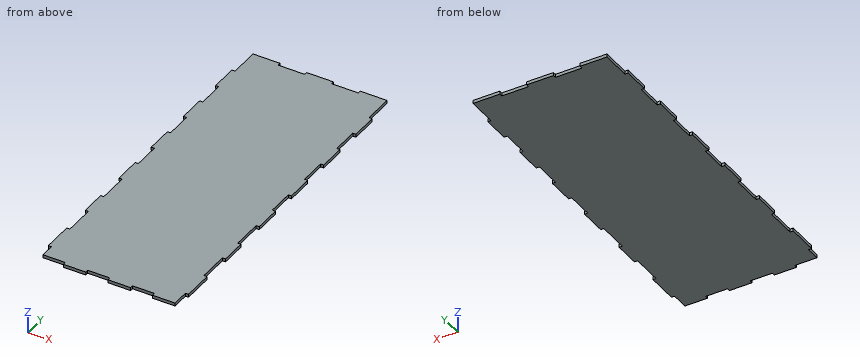
from build123d import *

# Parameters (mm, degrees)
BOSS_EXTRUDE1_DEPTH = 3


with BuildPart() as part:
    # Sketch1 → Boss-Extrude1 (new body)
    with BuildSketch(Plane.XY):
        Polygon((64.15, 153.019232641), (64.15, 178.481870793), (67.15, 178.481870793), (67.15, 204.244508944), (64.15, 204.244508944), (64.15, 229.707147096), (67.15, 229.707147096), (67.15, 255.469785247), (64.15, 255.469785247), (64.15, 280.932423398), (67.15, 280.932423398), (67.15, 306.69506155), (64.15, 306.69506155), (64.15, 335.261916889), (38.37, 335.261916889), (38.37, 332.261916889), (12.89, 332.261916889), (12.89, 335.261916889), (-12.89, 335.261916889), (-12.89, 332.261916889), (-38.37, 332.261916889), (-38.37, 335.261916889), (-64.15, 335.261916889), (-64.15, 306.69506155), (-67.15, 306.69506155), (-67.15, 280.932423398), (-64.15, 280.932423398), (-64.15, 255.469785247), (-67.15, 255.469785247), (-67.15, 229.707147096), (-64.15, 229.707147096), (-64.15, 204.244508944), (-67.15, 204.244508944), (-67.15, 178.481870793), (-64.15, 178.481870793), (-64.15, 153.019232641), (-67.15, 153.019232641), (-67.15, 127.25659449), (-64.15, 127.25659449), (-64.15, 98.12172779), (-67.15, 98.12172779), (-67.15, 73.67315636), (-64.15, 73.67315636), (-64.15, 44.27458493), (-67.15, 44.27458493), (-67.15, 14.8260135), (-64.15, 14.8260135), (-64.15, 1.5), (-42.916666667, 1.5), (-42.916666667, -1.5), (-21.383333333, -1.5), (-21.383333333, 1.5), (-0.15, 1.5), (-0.15, -1.5), (21.383333333, -1.5), (21.383333333, 1.5), (42.616666667, 1.5), (42.616666667, -1.5), (64.15, -1.5), (64.15, 14.8260135), (67.15, 14.8260135), (67.15, 44.27458493), (64.15, 44.27458493), (64.15, 73.67315636), (67.15, 73.67315636), (67.15, 98.12172779), (64.15, 98.12172779), (64.15, 127.25659449), (67.15, 127.25659449), (67.15, 153.019232641), align=None)
    extrude(amount=BOSS_EXTRUDE1_DEPTH)


solid = part.part
Can you work these out from the model? Positions are in its coordinate system, mm. Give positions to 0.01 mm unless a question says otherwise; leave off trailing zeros. Loops run counter-clockwise (first coordinate to the right, second up) from the corner with the lowest first, then second, coordinate; pieces in that order, holes last. Notation, with made-up numbers: (89.5, -12) -> (100.5, -12) arc R17 cw to (100.5, -3) -> close; hole circle Ø8 at (20.25, -17). An arc over 180 degrees is marked (long way). Use one line per item in the form item = value.
1) I need wall thicknesses on line 1 along Y through (x, z) = (-9, 2.7); line 2 along X through (y, z) = (262.5, 1.8); line 3 along Y through (x, z) = (-21.5, 1.5). Which ranges of each line are inside material? Lowest first, please.
Answers:
line_1 = 1.5 to 335.26
line_2 = -64.15 to 64.15
line_3 = -1.5 to 332.26
2) If we section it at A-A (x = -17): Please give me the cut outline in (y, z), plus the area to 3 significant figures.
Answers:
outline = (1.5, 0) -> (332.26, 0) -> (332.26, 3) -> (1.5, 3) -> close
area = 992 mm²
3) Will these pins go through, and if not, where does the flat tip stop? pin 1 (0.9 mm diameter, centred on x = -66, z = 2, fed in from -Y); pin 2 (1 mm diameter, centred on x = -43.5, z = 2, fed in from -Y); pin 3 (6 mm diameter, centred on x = 46.5, y = 126.5, fed in from -Z); pin 4 (0.9 mm diameter, centred on y = 66.5, z = 2, fed in from +X).
Answers:
pin_1 = 14.83
pin_2 = 1.5
pin_3 = 0
pin_4 = 64.15
4) If we section it at B-B (y = 209.5): Please give me the cut outline in (x, z), plus the area to 3 significant figures.
Answers:
outline = (-64.15, 0) -> (64.15, 0) -> (64.15, 3) -> (-64.15, 3) -> close
area = 385 mm²
